Verification items for the finished model (mm, model axes). A direction names the side the tool comes from. Give positions to 0.01 mm unless a question says otherwise; leave off trailing zeros. Order: outer loops, then holes, each group sorted by start corner. A loop starts at its lowest first (then second) coordinate and runs counter-clockwise, first axis right, second up. Notation, with made-up numbers: (-1.5, 63) -> (53.5, 63) arc R14 ccw to (53.5, 85) -> close; hole circle Ø11 at (13.5, -3.75). An arc over 180 degrees is marked (long way). Return JSON: item names as keys, results as strings. Group by question number.
(1) Tool access check on faces 1 (the face through (0, -15.875, 234)), 2 (the face through (-17, 0, -12.7)). Record the directions out of +Z, -Z, +X, -X, +Y, -Y that give a thin tool (end or side, any length) a straight path to the whole face; none if there is none.
(2) Depth check by flat-ended pin: pin 1 Ø4 at (x, y) = (7.5, 12.5) entering from +Z. Enter the tip coordinate at first touch or a pass-through.
(3) Thickness scan on line 1 along X through (y, z) = (2.5, 25.5) (3 decimals). Record the ranges inside material, lowest first.
(4) Cross-section at A-A on z = 84. Enter the section's corners in (x, y) (3 decimals).
(5) Release check for a two-part mould opening along X. For faces 3 (the face through (0, 19.05, 234)), 4 (the face through (15.875, 0, 234)), 5 (the face through (-19.05, 0, 234)) record: pulls with the +X half, pulls with the -X half, needs draft (parallel to the pull), parting line crosses it, or undercut.
Autodesk Inventor part; units mm, degrees
ref_plane "Start Plane" through (0, 0, -12.7) normal (0, 0, 1) x (1, 0, 0)
ref_plane "End Plane" through (0, 0, 487.3625) normal (0, 0, 1) x (1, 0, 0)
ref_plane "Work Plane6" through (762, 19.05, -12.7) normal (0, 0, -1) x (-1, 0, 0)
ref_plane "Start Plane" through (0, 0, -12.7) normal (0, 0, 1) x (1, 0, 0)
ref_plane "End Plane" through (0, 0, 487.3625) normal (0, 0, 1) x (1, 0, 0)
sketch "Sketch" plane through (0, 0, 0) normal (0, 0, 1) x (1, 0, 0)
  line L0 (-19.05, 19.05) -> (19.05, 19.05)
  line L1 (19.05, 19.05) -> (19.05, -19.05)
  line L2 (19.05, -19.05) -> (-19.05, -19.05)
  line L3 (-19.05, -19.05) -> (-19.05, 19.05)
  line L4 (15.875, 15.875) -> (-15.875, 15.875)
  line L5 (-15.875, 15.875) -> (-15.875, -15.875)
  line L6 (-15.875, -15.875) -> (15.875, -15.875)
  line L7 (15.875, -15.875) -> (15.875, 15.875)
  point P0 (0, 0)
  point P1 (0, 19.05)
  point P2 (-19.05, 0)
  dimension "width" = 38.1
  dimension "d1" = 3.175
extrude "Body" add sketch "Sketch" along normal up to surface (500.0625 mm away) from surface at -12.7
sketch "Sketch4" plane through (0, 0, 0) normal (0, 0, 1) x (1, 0, 0)
  line L0 (0, 0) -> (10, 0)
ref_plane "Work Plane4" through (0, 0, 0) normal (0, -1, 0) x (1, 0, 0)
sketch "Sketch5" plane through (0, 0, 0) normal (0, -1, 0) x (1, 0, 0)
  line L0 (-2, -12.7) -> (12, -12.7)
  line L1 (-2, 487.3625) -> (12, 487.3625)
  dimension "d9" = 500.0625
ref_plane "Work Plane6" through (762, 19.05, -12.7) normal (0, 0, -1) x (-1, 0, 0)
split "Split2" plane through (762, 19.05, -12.7) removes the side toward (0, 0, -1)
ref_plane "Work Plane7" through (38.1, 19.05, 487.3625) normal (0, 0, 1) x (1, 0, 0)
split "Split3" plane through (38.1, 19.05, 487.3625) removes the side toward (0, 0, 1)
equation "\"G_OFFSET_START\" = 12.7"
equation "\"G_OFFSET_END\" = -20.6375"
equation "\"d4\" = -G_OFFSET_START"
equation "\"d5\" = length + G_OFFSET_END"
equation "\"G_L\" = 812.8"
properties part number "1.5x1.5x.125 Tube" material "Aluminum-6061"
Verdict:
{
 "1": {"face 1": "+Z, -Z", "face 2": "-Z, +X, -X, +Y, -Y"},
 "2": {"pin 1": "through"},
 "3": {"line 1": "-19.05 to -15.875, 15.875 to 19.05"},
 "4": {"outline": "(-19.05, -19.05) -> (19.05, -19.05) -> (19.05, 19.05) -> (-19.05, 19.05) -> close; hole (-15.875, -15.875) -> (15.875, -15.875) -> (15.875, 15.875) -> (-15.875, 15.875) -> close"},
 "5": {"face 3": "needs draft", "face 4": "undercut", "face 5": "pulls with the -X half"}
}
